Could you check a few things on this model? Use its own coordinates, in mm. A direction names the side the tool comes from. Give positions to 0.01 mm unless a question says otherwise; leave off trailing zeros. Order: outer loops, then holes, each group sorted by start corner. A loop starts at its lowest first (then second) coordinate and runs counter-clockwise, first axis right, second up. Notation, with made-up numbers: (-1, 64.25) - (10, 64.25) arc R24 cw to (10, 76.25) - close; hole circle Ø5 at (-3.75, -18.75). An arc over 180 degrees is marked (long way). Put each result on its own line as item: value.
from build123d import *

# Parameters (mm, degrees)
F2_R     = 1.5875
F3_DEPTH = 12.701


with BuildPart() as f1:
    # F0 (on Right) → F1 (revolve)
    with BuildSketch(Plane.YZ):
        Polygon((0, 50.8), (0, 0), (12.7, 0), (12.7, 50.8), (8.382, 50.8), (8.382, 44.45), (4.318, 44.45), (4.318, 50.8), align=None)
    revolve(axis=Axis((0, 6.35, 0), (0, 1, 0)))

    # F2 (on face) → F3 (cut, through all)
    with BuildSketch(Plane.XZ):
        Circle(F2_R)
    extrude(amount=-F3_DEPTH, mode=Mode.SUBTRACT)


solid = f1.part
1) Suppose I cut it at C-C, the plane y = 2.25. List the corners of the cut face in (x, z) for me (1 decimal), and give its area (3 significant figures).
Filled in:
outline: circle Ø101.6 at (0, 0); hole circle Ø3.2 at (0, 0)
area: 8,100 mm^2
2) Suppose I cut it at B-B, the plane x = 0. List the corners of the cut face in (y, z) for me.
Filled in:
outline: (0, -50.8) - (4.32, -50.8) - (4.32, -44.45) - (8.38, -44.45) - (8.38, -50.8) - (12.7, -50.8) - (12.7, -1.59) - (0, -1.59) - close; (0, 1.59) - (12.7, 1.59) - (12.7, 50.8) - (8.38, 50.8) - (8.38, 44.45) - (4.32, 44.45) - (4.32, 50.8) - (0, 50.8) - close
3) Suppose I cut it at A-A, the plane z = 0. List the corners of the cut face in (x, y) for me, and give its area (3 significant figures).
Filled in:
outline: (-50.8, 0) - (-1.59, 0) - (-1.59, 12.7) - (-50.8, 12.7) - (-50.8, 8.38) - (-44.45, 8.38) - (-44.45, 4.32) - (-50.8, 4.32) - close; (1.59, 0) - (50.8, 0) - (50.8, 4.32) - (44.45, 4.32) - (44.45, 8.38) - (50.8, 8.38) - (50.8, 12.7) - (1.59, 12.7) - close
area: 1,200 mm^2
4) I'm going to push flat-ended pins straight in: pin 1 (1 mm diameter, centred on x = -5, y = 10.5, fed in from +Z); pin 2 (5 mm diameter, centred on x = 0, z = 0, fed in from -Y); pin 3 (1.5 mm diameter, centred on x = 10, y = 11, fed in from +Z); pin 4 (1.5 mm diameter, centred on x = 8, y = 5.5, fed in from +Z). Where does each tip first touch, or does it pass through?
Filled in:
pin 1: stops at z = 50.6
pin 2: stops at y = 0
pin 3: stops at z = 49.95
pin 4: stops at z = 43.85
5) Suppose I cut it at D-D, the plane z = 33.5. List the corners of the cut face in (x, y) for me, and give its area (3 significant figures).
Filled in:
outline: (-38.19, 0) - (38.19, 0) - (38.19, 4.32) - (29.22, 4.32) - (29.22, 8.38) - (38.19, 8.38) - (38.19, 12.7) - (-38.19, 12.7) - (-38.19, 8.38) - (-29.22, 8.38) - (-29.22, 4.32) - (-38.19, 4.32) - close
area: 897 mm^2
6) We'd pull the mould along Z, two halves only. Please class faces 1 (the flat face through (1, 0, 11)), 2 (the cylindrical face through (-49.592, 2.129, -11.012)), 3 (the cylindrical face through (-0.34, 6.26, -1.55)): pulls with the +Z half, pulls with the -Z half, needs draft (parallel to the pull), parting line crosses it, or undercut.
Filled in:
face 1: needs draft
face 2: parting line crosses it
face 3: undercut
7) Which directions (+Z, -Z, +X, -X, +Y, -Y) give clear straight access to the entire face, cutting with the end or side of a thin tool? Please do faces 4 (the cylindrical face through (-49.592, 10.511, -11.012)), 5 (the cylindrical face through (13.352, 6.322, 42.397)).
Filled in:
face 4: +Y, -Y
face 5: none
8) If I drill on line 1 (Y direction, x = -44, z = -9.5); line 2 (X direction, y = 12.25, z = 7.5); line 3 (Z direction, x = 4.5, y = 1.5), over which ranges is the centre line in solid material (lowest first)? Write a range as [from, to].
Filled in:
line 1: y = [0, 4.32], [8.38, 12.7]
line 2: x = [-50.24, 50.24]
line 3: z = [-50.6, 50.6]
